from build123d import *

# Parameters (mm, degrees)
SKETCH_1_R      = 1.5
SKETCH_1_R_2    = 2
EXTRUDE_1_DEPTH = 3


with BuildPart() as part:
    # 草图1 → 凸台-拉伸1 (new body)
    with BuildSketch(Plane.XY):
        with BuildLine():
            Line((-2.286729251, -0.246717108), (-3.883861716, 14.556510567))
            ThreePointArc((-3.883861716, 14.556510567), (-3.854723084, 14.925691914), (-3.693228018, 15.258953478))
            ThreePointArc((-3.693228018, 15.258953478), (-0.747195178, 24.211667814), (-3.723167614, 33.154474505))
            ThreePointArc((-3.723167614, 33.154474505), (-3.872965508, 33.444371631), (-3.921458744, 33.767060581))
            Line((-3.921458744, 33.767060581), (-3.069651306, 91.604785634))
            ThreePointArc((-3.069651306, 91.604785634), (-0.067427131, 94.551575772), (2.911665375, 91.581402384))
            Line((2.911665375, 91.581402384), (3.267124799, 40.124176415))
            ThreePointArc((3.267124799, 40.124176415), (3.324280751, 39.797782311), (3.484958279, 39.507984717))
            ThreePointArc((3.484958279, 39.507984717), (8.841844113, 24.158825584), (3.450331122, 8.821795246))
            ThreePointArc((3.450331122, 8.821795246), (3.307226898, 8.579714374), (3.237181652, 8.307362338))
            Line((3.237181652, 8.307362338), (2.285932959, -0.25398919))
            ThreePointArc((2.285932959, -0.25398919), (-0.003657774, -2.299997091), (-2.286729251, -0.246717108))
        make_face()
        with Locations((-0.07911944, 91.560742455)):
            Circle(SKETCH_1_R, mode=Mode.SUBTRACT)
        with Locations((-0.073800571, 13.899599644)):
            Circle(SKETCH_1_R, mode=Mode.SUBTRACT)
        with Locations((0, 1)):
            Circle(SKETCH_1_R_2, mode=Mode.SUBTRACT)
    extrude(amount=EXTRUDE_1_DEPTH)


solid = part.part
Verification items for the finished model (mm, model axes). Round coordinates to 2 decimals unless told otherwise and drop trailing zeros. Order: outer loops, then holes, each group sorted by start corner. A loop starts at its lowest first (then second) coordinate and runs counter-clockwise, first axis right, second up.
1. Release check for a two-part mould opening along Y. For faces 1 (the cylindrical face through (-0.748, 24.077, 1.479)), 2 (the cylindrical face through (-0.13, 94.55, 1.48)), 3 (the cylindrical face through (8.84, 24.39, 1.48)) record: +Y half, -Y half, draft (parallel to the pull), parting line (faces both ways), or undercut.
Final values:
face 1: undercut
face 2: +Y half
face 3: parting line
2. Go/stop test with flat-tipped pins: P1, Ø1.8, axis at x = -0.07, y = 13.9, coming from the -Z side; P2, Ø1, axis at x = -1.5, z = 1.5, coming from the +Y side. Record where each tip stops, or that it passes through.
Final values:
P1: passes through
P2: stops at y = 94.41
3. Section check B-B on y = 1. Record the cut outline in (x, z).
Final values:
outline: (-2.42, 0) - (-2, 0) - (-2, 3) - (-2.42, 3) - close; (2, 0) - (2.43, 0) - (2.43, 3) - (2, 3) - close
4. Section check D-D on y = 76. Record the cut outline in (x, z).
Final values:
outline: (-3.3, 0) - (3.02, 0) - (3.02, 3) - (-3.3, 3) - close
5. Section check C-C on y = 32. Record the cut outline in (x, z), then the cut area to 3 significant figures.
Final values:
outline: (-2.94, 0) - (7.57, 0) - (7.57, 3) - (-2.94, 3) - close
area: 31.5 mm2
6. Section check A-A on z = 0.9. Record the cut outline in (x, y).
Final values:
outline: (-3.92, 33.77) arc R1 ccw to (-3.72, 33.15) arc R15 cw to (-3.69, 15.26) arc R1 ccw to (-3.88, 14.56) - (-2.29, -0.25) arc R2.3 ccw to (2.29, -0.25) - (3.24, 8.31) arc R1 cw to (3.45, 8.82) arc R24.59 ccw to (3.48, 39.51) arc R1 cw to (3.27, 40.12) - (2.91, 91.58) arc R2.99 ccw to (-3.07, 91.6) - close; hole circle Ø4 at (0, 1); hole circle Ø3 at (-0.08, 91.56); hole circle Ø3 at (-0.07, 13.9)
7. Thickness scan on L1, parallel to Y at x = 0, z = 1.25; L2, parallel to Y at x = 0.75, z = 2.7; L3, parallel to X at y = 46, z = 1.9. Record the ranges inside material, lowest first.
Final values:
L1: y = -2.3 to -1, 3 to 12.4, 15.4 to 90.06, 93.06 to 94.55
L2: y = -2.17 to -0.85, 2.85 to 12.65, 15.15 to 90.31, 92.81 to 94.43
L3: x = -3.74 to 3.23
